Check sheet for the modelled part. Datum: model origin and axes. Units: mm. Face numbers are marked on the shaded views. A direction names the side the tool comes from. Give positions to 0.01 mm unless a question says otherwise; leave off trailing zeros. Write each loop counter-clockwise with the first axis right and the second up, starting at its lowest first coordinate (ties: lowest second). Pieces come first, ordered by that corner, then holes. Notation, with made-up numbers: (79, 11.25) -> (131, 11.25) arc R11 cw to (131, 26.25) -> close; hole circle Ø9 at (58, -3). An arc over 180 degrees is marked (long way). Answer as a JSON object with one key per item and string values.
from build123d import *

# Parameters (mm, degrees)
BOSS_EXTRUDE1_DEPTH = 5


with BuildPart() as part:
    # Sketch2 → Boss-Extrude1 (new body)
    with BuildSketch(Plane.XY):
        with BuildLine():
            Line((-1.4, 7.8), (1.4, 7.8))
            Line((1.4, 7.8), (1.4, 5.2))
            ThreePointArc((1.4, 5.2), (1.329474497, 4.681174375), (1.123016035, 4.2))
            ThreePointArc((1.123016035, 4.2), (0.84603207, 3.2), (1.123016035, 2.2))
            ThreePointArc((1.123016035, 2.2), (1.329474497, 1.718825625), (1.4, 1.2))
            Line((1.4, 1.2), (1.4, -1.4))
            ThreePointArc((1.4, -1.4), (1.253553391, -1.753553391), (0.9, -1.9))
            ThreePointArc((0.9, -1.9), (0.546446609, -2.046446609), (0.4, -2.4))
            ThreePointArc((0.4, -2.4), (0.546446609, -2.753553391), (0.9, -2.9))
            Line((0.9, -2.9), (2.3, -2.9))
            ThreePointArc((2.3, -2.9), (2.653553391, -2.753553391), (2.8, -2.4))
            Line((2.8, -2.4), (2.8, 1.2))
            ThreePointArc((2.8, 1.2), (2.729474497, 1.718825625), (2.523016035, 2.2))
            ThreePointArc((2.523016035, 2.2), (2.24603207, 3.2), (2.523016035, 4.2))
            ThreePointArc((2.523016035, 4.2), (2.729474497, 4.681174375), (2.8, 5.2))
            Line((2.8, 5.2), (2.8, 8.2))
            ThreePointArc((2.8, 8.2), (2.507106781, 8.907106781), (1.8, 9.2))
            Line((1.8, 9.2), (-1.8, 9.2))
            ThreePointArc((-1.8, 9.2), (-2.507106781, 8.907106781), (-2.8, 8.2))
            Line((-2.8, 8.2), (-2.8, 5.2))
            ThreePointArc((-2.8, 5.2), (-2.729474497, 4.681174375), (-2.523016035, 4.2))
            ThreePointArc((-2.523016035, 4.2), (-2.24603207, 3.2), (-2.523016035, 2.2))
            ThreePointArc((-2.523016035, 2.2), (-2.729474497, 1.718825625), (-2.8, 1.2))
            Line((-2.8, 1.2), (-2.8, -2.4))
            ThreePointArc((-2.8, -2.4), (-2.653553391, -2.753553391), (-2.3, -2.9))
            Line((-2.3, -2.9), (-0.9, -2.9))
            ThreePointArc((-0.9, -2.9), (-0.546446609, -2.753553391), (-0.4, -2.4))
            ThreePointArc((-0.4, -2.4), (-0.546446609, -2.046446609), (-0.9, -1.9))
            ThreePointArc((-0.9, -1.9), (-1.253553391, -1.753553391), (-1.4, -1.4))
            Line((-1.4, -1.4), (-1.4, 1.2))
            ThreePointArc((-1.4, 1.2), (-1.329474497, 1.718825625), (-1.123016035, 2.2))
            ThreePointArc((-1.123016035, 2.2), (-0.84603207, 3.2), (-1.123016035, 4.2))
            ThreePointArc((-1.123016035, 4.2), (-1.329474497, 4.681174375), (-1.4, 5.2))
            Line((-1.4, 5.2), (-1.4, 7.8))
        make_face()
    extrude(amount=BOSS_EXTRUDE1_DEPTH)


solid = part.part
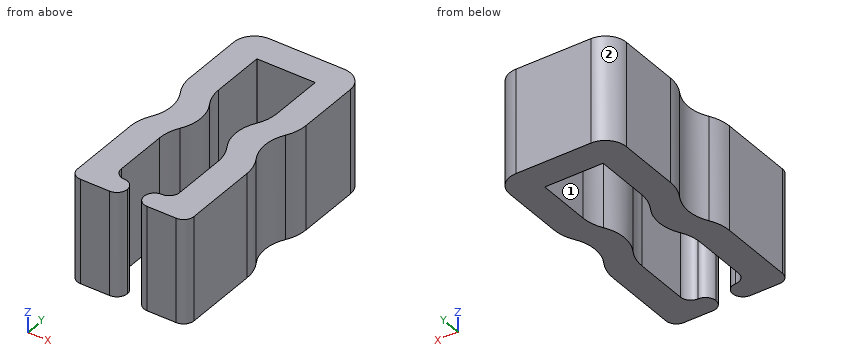
1. Sectioned sample at C-C, the plane x = 1.25. Enter the section's corners in (y, z).
Determined:
{"outline": "(-2.9, 0) -> (-1.76, 0) -> (-1.76, 5) -> (-2.9, 5) -> close; (1.95, 0) -> (4.45, 0) -> (4.45, 5) -> (1.95, 5) -> close; (7.8, 0) -> (9.2, 0) -> (9.2, 5) -> (7.8, 5) -> close"}
2. Sectioned sample at D-D, the plane x = 0.1. Enter the section's corners in (y, z).
Determined:
{"outline": "(7.8, 0) -> (9.2, 0) -> (9.2, 5) -> (7.8, 5) -> close"}
3. Scan lines: L1, parallel to X at y = 7.75, z = 4.5; L2, parallel to X at y = 3.25, z = 2.25; L3, parallel to Y at x = 0.5, z = 2.15. Record each from-to range of solid material in increasing order. Write a range as [from, to].
Determined:
{"L1": "[-2.8, -1.4], [1.4, 2.8]", "L2": "[-2.25, -0.85], [0.85, 2.25]", "L3": "[-2.7, -2.1], [7.8, 9.2]"}
4. Access from +Z, -Z, +X, -X, +Y, -Y to the whole of each face (thin tool, end or side, straight path). Record for the marked faces 1 and 2.
Determined:
{"face 1": "+Z, -Z", "face 2": "+Z, -Z, -X, +Y"}
5. Sectioned sample at A-A, the plane y = -1. Enter the section's corners in (x, z).
Determined:
{"outline": "(-2.8, 0) -> (-1.4, 0) -> (-1.4, 5) -> (-2.8, 5) -> close; (1.4, 0) -> (2.8, 0) -> (2.8, 5) -> (1.4, 5) -> close"}
6. Go/stop test with a flat-tipped pin: P1, Ø1.5, axis at y = 2, z = 2, coming from the +X side. Record where the tip stops, or that it passes through.
Determined:
{"P1": "x = 2.8"}
